Source: CAD feature listing. Evaluate the final solid. Frame: model axes, mm. Give positions to 0.01 mm unless a question says otherwise; leave off trailing zeros. Order: outer loops, then holes, each group sorted by start corner. A loop starts at its lowest first (then second) coordinate and runs counter-clockwise, first axis right, second up. Notation, with made-up numbers: (-35, 4) - (16, 4) arc R17 cw to (16, 30) - close; hole circle Ø7 at (77, 30.5). An arc over 180 degrees is marked (long way). Write each question's results on one line, items separated by ' | '. Start each with the question number.
Item 1: Line query: line 1 along Z through (x, y) = (-4, -0.25); line 2 along Z through (x, y) = (-31, -2.25); line 3 along X through (y, z) = (-2.1, 53.5). Output: solid intervals per line, ascending.
Item 2: Mould query, pull axis X, two halves, no side actions, for faces 1 (the cylindrical face through (-10.64, -0.74, 242.9)), 2 (the flat face through (-3, -2.5, 240)), 3 (the cylindrical face through (-10.64, -0.74, 32.9)). Classes: released by +X, released by -X, zero draft, split by the parting line, or undercut.
Item 3: Section B-B on x = 8. State how many separate pieces and enclosed holes the cut face has, and give its area (3 significant figures).
Item 4: Section A-A on y = -2.1. Output: boundary loops of the cut face in (x, z).
```python
from build123d import *

# Parameters (mm, degrees)
F0_W     = 92
F0_H     = 554
F0_R     = 38
F1_DEPTH = 2.5
F2_SIZE  = 1


with BuildPart() as f1:
    # F0 (on Front) → F1 (new body)
    with BuildSketch(Plane.XZ):
        with Locations((-2.399907, 174.997145)):
            Rectangle(F0_W, F0_H)
        with Locations((-2.399907, -35.002855)):
            Circle(F0_R, mode=Mode.SUBTRACT)
        with Locations((-2.399907, 69.997145)):
            Circle(F0_R, mode=Mode.SUBTRACT)
        with Locations((-2.399907, 174.997145)):
            Circle(F0_R, mode=Mode.SUBTRACT)
        with Locations((-2.399907, 279.997145)):
            Circle(F0_R, mode=Mode.SUBTRACT)
        with Locations((-2.399907, 384.997145)):
            Circle(F0_R, mode=Mode.SUBTRACT)
    extrude(amount=F1_DEPTH)

    # F2
    f2_edges = [f1.edges().sort_by_distance(p)[0] for p in [
        (-2.399907, -2.5, -102.002855),
        (43.600093, -2.5, 174.997145),
        (-2.399907, -2.5, 451.997145),
        (-48.399907, -2.5, 174.997145),
        (-40.399907, -2.5, -35.002855),
        (-40.399907, -2.5, 69.997145),
        (-40.399907, -2.5, 174.997145),
        (-40.399907, -2.5, 279.997145),
        (-40.399907, -2.5, 384.997145),
    ]]
    chamfer(f2_edges, length=F2_SIZE)


solid = f1.part
```
Evaluation:
1) line 1: z = -102 to -72.97, 2.96 to 32.03, 107.96 to 137.03, 212.96 to 242.03, 317.96 to 347.03, 422.96 to 452 | line 2: z = -101.25 to -61.15, -8.86 to 43.85, 96.14 to 148.85, 201.14 to 253.85, 306.14 to 358.85, 411.14 to 451.25 | line 3: x = -47.8 to -37.3, 32.5 to 43
2) face 1: undercut | face 2: zero draft | face 3: undercut
3) separate pieces: 6 | enclosed holes: 0 | area: 465 mm^2
4) outline: (-47.8, -101.4) - (43, -101.4) - (43, 451.4) - (-47.8, 451.4) - close; hole circle Ø77.2 at (-2.4, -35); hole circle Ø77.2 at (-2.4, 70); hole circle Ø77.2 at (-2.4, 175); hole circle Ø77.2 at (-2.4, 280); hole circle Ø77.2 at (-2.4, 385)
